from build123d import *

# Parameters (mm, degrees)
F0_R      = 9.525
F1_DEPTH  = 12.7
F2_R      = 6.6675
F3_DEPTH  = 9.525
F4_W      = 1.1684
F4_H      = 2.2352
F6_R      = 8.636
F7_DEPTH  = 10
F8_R      = 4.9
F9_DEPTH  = 2.5
F10_R     = 2.5
F11_DEPTH = 25.4
F12_R     = 3.5
F13_DEPTH = 2
F14_SIZE  = 0.6


with BuildPart() as f1:
    # F0 (on Top) → F1 (new body)
    with BuildSketch(Plane.XY):
        Circle(F0_R)
    extrude(amount=F1_DEPTH)

    # F2 (on face) → F3 (cut)
    with BuildSketch(Plane.XY.offset(12.7)):
        Circle(F2_R)
    extrude(amount=-F3_DEPTH, mode=Mode.SUBTRACT)

    # F4 (on Front) → F5 (revolve, cut)
    with BuildSketch(Plane.XZ):
        with Locations((7.2517, 9.9949)):
            Rectangle(F4_W, F4_H)
    revolve(axis=Axis((0, 0, 19.022157), (0, 0, 1)), mode=Mode.SUBTRACT)

    # F6 (on face) → F7 (join)
    with BuildSketch(Plane(origin=(0, 0, 0), x_dir=(1, 0, 0), z_dir=(0, 0, -1))):
        Circle(F6_R)
    extrude(amount=F7_DEPTH)

    # F8 (on face) → F9 (cut)
    with BuildSketch(Plane(origin=(0, 0, -10), x_dir=(1, 0, 0), z_dir=(0, 0, -1))):
        Circle(F8_R)
    extrude(amount=-F9_DEPTH, mode=Mode.SUBTRACT)

    # F10 (on face) → F11 (cut)
    with BuildSketch(Plane.XY.offset(3.175)):
        Circle(F10_R)
    extrude(amount=-F11_DEPTH, mode=Mode.SUBTRACT)

    # F12 (on face) → F13 (cut)
    with BuildSketch(Plane(origin=(0, 0, -7.5), x_dir=(1, 0, 0), z_dir=(0, 0, -1))):
        Circle(F12_R)
    extrude(amount=-F13_DEPTH, mode=Mode.SUBTRACT)

    # F14
    f14_edges = [f1.edges().sort_by_distance(p)[0] for p in [
        (-4.9, 0, -10),
        (-8.636, 0, -10),
    ]]
    chamfer(f14_edges, length=F14_SIZE)


solid = f1.part
Input: part model. Units: mm. Frame: model coordinates. A direction names the side the tool comes from. Coordinates: 2 decimals unless noted, no trailing zeros. Loops run counter-clockwise (first coordinate to the right, second up) from the corner with the lowest first, then second, coordinate; pieces in that order, holes last. Notation, with made-up numbers: (-33, -33.75) -> (10, -33.75) arc R28 cw to (10, 2.25) -> close; hole circle Ø8 at (-39, -27). An arc over 180 degrees is marked (long way). Write each question's results on one line, items separated by ' | '. Start each with the question number.
Q1. Section B-B, the plane z = 0.5. Return the cut outline in (x, y) (3 decimals).
Q2. Reachability of faces 4 (the cylindrical face through (-1.7, -7.65, 10.01)), 5 (the cylindrical face through (-0.54, -2.44, -1.1)), 6 (the flat face through (2.1, 3.2, -7.5)), 7 (the flat face through (-2.3, 6.5, 12.7)), 8 (the cylindrical face through (-0.87, 6.61, 6.07)) from +Z, -Z, +X, -X, +Y, -Y: full face, straight path, thin tool, end or side. Return the list, or none.
Q3. Ray query, line 1 (Z direction, x = -5.5, y = -4.5); line 2 (Y direction, x = 0, z = -8.55); line 3 (X direction, y = 0, z = -7.05). Return the intervals inside material, ascending. Write a range as from..to.
Q4. Pin query (flat end, axial travel): pin 1 (8 mm diameter, centred on x = 0, y = 0, fed in from -Z); pin 2 (7.5 mm diameter, centred on x = 1, y = -1, fed in from -Z); pin 3 (1.5 mm diameter, centred on x = -6.5, z = 4.5, fed in from -Y). Return the tip coordinate at first contact, or that it passes through.
Q5. Pull-direction query (Y, two-part tool) for faces 1 (the flat face through (3, 5, -10)), 2 (the cylindrical face through (-1.124, -8.563, -4.634)), 3 (the cylindrical face through (-1.062, 4.783, -8.463)); classes: released by +Y, released by -Y, zero draft, split by the parting line, or undercut.
Found:
1) outline: circle Ø19.05 at (0, 0); hole circle Ø5 at (0, 0)
2) face 4: none | face 5: +Z, -Z | face 6: -Z | face 7: +Z, +X, -X, +Y, -Y | face 8: +Z
3) line 1: -10..8.88, 11.11..12.7 | line 2: -8.64..-4.9, 4.9..8.64 | line 3: -8.64..-3.5, 3.5..8.64
4) pin 1: z = -7.5 | pin 2: z = -9.66 | pin 3: y = -7.59
5) face 1: zero draft | face 2: split by the parting line | face 3: undercut
